Build history of the part. All positions in model axes, mm. Face numbers are marked on the shaded views. A direction names the side the tool comes from. Give positions to 0.01 mm unless a question says otherwise; leave off trailing zeros. Order: outer loops, then holes, each group sorted by start corner. A loop starts at its lowest first (then second) coordinate and runs counter-clockwise, first axis right, second up. Notation, with made-up numbers: (45, 86.25) - (103, 86.25) arc R11 ccw to (103, 95.25) - close; hole circle Ø3 at (-24, 15.25). An arc over 180 degrees is marked (long way). Write each question's results on one line, items separated by ' | '. Start each with the question number.
1) Tool access for the marked faces 5 and 6: list every direction of +Z, -Z, +X, -X, +Y, -Y with a clear straight run to the whole face (end or side of a thin tool).
2) Drop a flat-ended pin along its axis: pin 1 Ø3.5 at (y, z) = (0, 5) entering from -X. Give the stop position or say it passes through.
3) Drill centre lines: line 1 along Y through (x, z) = (-1, 61.5); line 2 along Y through (x, z) = (-4.7, 5). Where is each one in solid material? Low to high. Write a range as from..to.
4) Two-plate mould, pull along X, no slides. Class the marked faces 1, 2, 3 and 4: +X half, -X half, draft (parallel to the pull), parting line (faces both ways), or undercut.
5) Cut at B-B on y = -2.5. List the corners of the cut face in (x, z).
6) Cut at D-D on z = 63. List the corners of the cut face in (x, y), plus the area to 3 significant figures.
7) Cut at A-A on z = 5. List the corners of the cut face in (x, y).
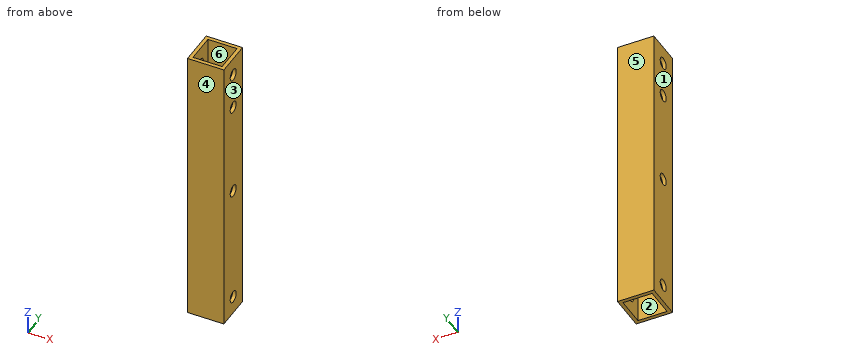
from build123d import *

# Parameters (mm, degrees)
SKETCH_1_W          = 10
SKETCH_1_H          = 10
SKETCH_1_W_2        = 8
SKETCH_1_H_2        = 8
EXTRUDE_1_DEPTH     = 78.81860214
SKETCH_2_R          = 1.6
CUT_EXTRUDE_1_DEPTH = 80.607612973
SKETCH_3_R          = 1.6
CUT_EXTRUDE_3_DEPTH = 80.607612973


with BuildPart() as part:
    # ｽｹｯﾁ1 → ﾎﾞｽ - 押し出し1 (new body)
    with BuildSketch(Plane.XY):
        Rectangle(SKETCH_1_W, SKETCH_1_H)
        Rectangle(SKETCH_1_W_2, SKETCH_1_H_2, mode=Mode.SUBTRACT)
    extrude(amount=EXTRUDE_1_DEPTH)

    # ｽｹｯﾁ2 → ｶｯﾄ - 押し出し1 (cut, through all)
    with BuildSketch(Plane(origin=(5, 0, 0), x_dir=(0, 0, -1), z_dir=(1, 0, 0))):
        with Locations((-5, 0)):
            Circle(SKETCH_2_R)
        with Locations((-73.81860214, 0)):
            Circle(SKETCH_2_R)
    extrude(amount=-CUT_EXTRUDE_1_DEPTH, mode=Mode.SUBTRACT)

    # ｽｹｯﾁ3 → ｶｯﾄ - 押し出し3 (cut, through all)
    with BuildSketch(Plane.ZY.offset(5)):
        with Locations((63.81860214, 0)):
            Circle(SKETCH_3_R)
        with Locations((37.81860214, 0)):
            Circle(SKETCH_3_R)
    extrude(amount=-CUT_EXTRUDE_3_DEPTH, mode=Mode.SUBTRACT)


solid = part.part
Results:
1) face 5: +Z, -Z, +X, -X, +Y | face 6: +Z, -Z
2) pin 1: x = -5
3) line 1: -5..-4, 4..5 | line 2: -5..-1.6, 1.6..5
4) face 1: -X half | face 2: undercut | face 3: +X half | face 4: draft
5) outline: (-5, 0) - (-4, 0) - (-4, 78.82) - (-5, 78.82) - close; (4, 0) - (5, 0) - (5, 78.82) - (4, 78.82) - close
6) outline: (-5, -5) - (5, -5) - (5, -1.37) - (4, -1.37) - (4, -4) - (-4, -4) - (-4, -1.37) - (-5, -1.37) - close; (-5, 1.37) - (-4, 1.37) - (-4, 4) - (4, 4) - (4, 1.37) - (5, 1.37) - (5, 5) - (-5, 5) - close | area: 30.5 mm^2
7) outline: (-5, -5) - (5, -5) - (5, -1.6) - (4, -1.6) - (4, -4) - (-4, -4) - (-4, -1.6) - (-5, -1.6) - close; (-5, 1.6) - (-4, 1.6) - (-4, 4) - (4, 4) - (4, 1.6) - (5, 1.6) - (5, 5) - (-5, 5) - close
